from build123d import *

# Parameters (mm, degrees)
F0_W     = 51.9770644605
F0_H     = 64.5220279694
F1_DEPTH = 25
F1_TAPER = 45
F2_R     = 4.0319564515
F3_DEPTH = 25


with BuildPart() as f1:
    # F0 (on Top) → F1 (new body)
    with BuildSketch(Plane.XY):
        with Locations((25.9885322303, 32.2610139847)):
            Rectangle(F0_W, F0_H)
    extrude(amount=F1_DEPTH, taper=F1_TAPER)

    # F2 (on face) → F3 (cut)
    with BuildSketch(Plane(origin=(25.9885322303, 0, 25.9885322303), x_dir=(0, 1, 0), z_dir=(0.7071067812, 0, 0.7071067812))):
        with Locations((35.5320125818, -18.2061810046)):
            Circle(F2_R)
    extrude(amount=-F3_DEPTH, mode=Mode.SUBTRACT)


solid = f1.part
Design review of the part built by this model. Coordinates are the model's own, in mm. Round coordinates to 2 decimals unless told otherwise and drop trailing zeros. Loops run counter-clockwise (first coordinate to the right, second up) from the corner with the lowest first, then second, coordinate; pieces in that order, holes last. Notation, with made-up numbers: M -18,-26 L 20,-26 A33 ccw 20,10 Z; hole C -22,2.25 d6. An arc over 180 degrees is marked long. Answer as a JSON object with one key per item and string values.
Item 1: We need section A-A on y = 32.5. Give the boundary of the cut face in (x, z).
Answer sheet:
{"outline": "M 0,0 L 21.99,0 L 36.98,14.99 L 26.98,25 L 25,25 Z; M 29.51,0 L 51.98,0 L 40.74,11.24 Z"}
Item 2: We need section B-B on z = 17.5. Give the boundary of the cut face in (x, y).
Answer sheet:
{"outline": "M 17.5,17.5 L 34.48,17.5 L 34.48,47.02 L 17.5,47.02 Z"}
Item 3: We need section C-C on y = 61.5. Give the boundary of the cut face in (x, z), and give its area (3 significant figures).
Answer sheet:
{"outline": "M 0,0 L 51.98,0 L 48.96,3.02 L 3.02,3.02 Z", "area": "148 mm^2"}
Item 4: Clearance check with flat-ended pins moving along their axes: P1, Ø1, axis at x = 18.5, y = 9.5, coming from the +Z side; P2, Ø6, axis at y = 18.5, z = 15, coming from the +X side; P3, Ø10, axis at x = 39, z = 18.5, coming from the -Y side. State where each tip first meets the part, or that it passes through.
Answer sheet:
{"P1": "stops at z = 10", "P2": "stops at x = 39.98", "P3": "stops at y = 13.53"}
Item 5: Wall thickness on L1, parallel to X at y = 32.5, z = 4.75; L2, parallel to Y at x = 36, z = 13; L3, parallel to Y at x = 23, z = 8: over which ranges is each line inside the solid? List them lowest first. Write a range as from..to.
Answer sheet:
{"L1": "x = 4.75..26.74, 34.26..47.23", "L2": "y = 13..32, 39.07..51.52", "L3": "y = 8..56.52"}
Item 6: The part is to be moulded in two halves that separate along Z. For faces 1 (the cylindrical face through (29.938, 35.007, 9.844)), 2 (the flat face through (31, 33, 0)), 3 (the flat face through (10, 32, 10)), say which applies: pulls with the +Z half, pulls with the -Z half, needs draft (parallel to the pull), parting line crosses it, or undercut.
Answer sheet:
{"face 1": "undercut", "face 2": "pulls with the -Z half", "face 3": "pulls with the +Z half"}
